```python
from build123d import *

# Parameters (mm, degrees)
SKETCH1_W           = 144
SKETCH1_H           = 331
BOSS_EXTRUDE1_DEPTH = 3
SKETCH2_R           = 5
CUT_EXTRUDE1_DEPTH  = 543.073379748
SKETCH3_R           = 5
CUT_EXTRUDE2_DEPTH  = 10
SKETCH4_R           = 5
CUT_EXTRUDE3_DEPTH  = 10
LPATTERN1_COUNT     = 4
LPATTERN1_PITCH     = 80
FILLET1_R           = 5


with BuildPart() as part:
    # Sketch1 → Boss-Extrude1 (new body)
    with BuildSketch(Plane.XY.offset(3)):
        with Locations((18.851179955, 368.89742901)):
            Rectangle(SKETCH1_W, SKETCH1_H)
    extrude(amount=-BOSS_EXTRUDE1_DEPTH)

    # Sketch2 → Cut-Extrude1 (cut, through all)
    with BuildSketch(Plane.XY.offset(3)):
        with Locations((63.851179955, 523.39742901)):
            Circle(SKETCH2_R)
        with Locations((64.635907686, 483.39742901)):
            Circle(SKETCH2_R)
        with Locations((64.635907686, 425.89742901)):
            Circle(SKETCH2_R)
        with Locations((64.635907686, 320.89742901)):
            Circle(SKETCH2_R)
        with Locations((64.635907686, 263.39742901)):
            Circle(SKETCH2_R)
        with Locations((64.635907686, 223.39742901)):
            Circle(SKETCH2_R)
    extrude(amount=-CUT_EXTRUDE1_DEPTH, mode=Mode.SUBTRACT)

    # Sketch3 → Cut-Extrude2 (cut)
    with BuildSketch(Plane.XY.offset(3)):
        with Locations((-26.148820045, 505.89742901)):
            Circle(SKETCH3_R)
        with Locations((-26.148820045, 400.89742901)):
            Circle(SKETCH3_R)
        with Locations((-26.148820045, 345.89742901)):
            Circle(SKETCH3_R)
        with Locations((-26.148820045, 240.89742901)):
            Circle(SKETCH3_R)
    extrude(amount=-CUT_EXTRUDE2_DEPTH, mode=Mode.SUBTRACT)

    # Sketch4 → Cut-Extrude3 (cut)
    with BuildSketch(Plane.XY.offset(3)):
        with Locations((-41.648820045, 253.39742901)):
            Circle(SKETCH4_R)
        with Locations((-11.148820045, 253.39742901)):
            Circle(SKETCH4_R)
        with Locations((48.851179955, 253.39742901)):
            Circle(SKETCH4_R)
        with Locations((79.351179955, 253.39742901)):
            Circle(SKETCH4_R)
    cut_extrude3 = extrude(amount=-CUT_EXTRUDE3_DEPTH, mode=Mode.SUBTRACT)

    # LPattern1: Cut-Extrude3 ×4
    with Locations(*[(0, i * LPATTERN1_PITCH, 0) for i in range(1, LPATTERN1_COUNT)]):
        add(cut_extrude3, mode=Mode.SUBTRACT)

    # Fillet1
    fillet1_edges = [part.edges().sort_by_distance(p)[0] for p in [
        (-53.148820045, 534.39742901, 1.5),
        (90.851179955, 534.39742901, 1.5),
    ]]
    fillet(fillet1_edges, radius=FILLET1_R)


solid = part.part
```
Can you work these out from the model? Positions are in its coordinate system, mm. Round coordinates to 2 decimals unless told otherwise and drop trailing zeros. Answer in a Markdown table with one row per item.
Item 1: Will this pin go through, and if not, where does the flat tip stop? P1, Ø6, axis at x = -11.15, y = 253.4, coming from the +Z side (3 decimals).
Answer block:
| item | result |
|---|---|
| P1 | through |
Item 2: Suppose I cut it at A-A, the plane z = 0.5. Give the number of separate pieces and of enclosed holes in the cut face, plus the area to 3 significant figures.
Answer block:
| item | result |
|---|---|
| separate pieces | 1 |
| enclosed holes | 26 |
| area | 45,600 mm² |
Item 3: If I drill on probe 1 along Y at (x, z) = (51, 2.25); probe 2 along Y at (x, z) = (48, 2.65); probe 3 along X at (y, z) = (259, 0.25), over which ranges is the centre line in solid material (lowest first)?
Answer block:
| item | result |
|---|---|
| probe 1 | 203.4 to 248.88, 257.91 to 328.88, 337.91 to 408.88, 417.91 to 488.88, 497.91 to 534.4 |
| probe 2 | 203.4 to 248.47, 258.32 to 328.47, 338.32 to 408.47, 418.32 to 488.47, 498.32 to 534.4 |
| probe 3 | -53.15 to 62.26, 67.02 to 90.85 |
Item 4: We'd pull the mould along Y, two halves only. Please class faces 1 (the flat face through (18, 371, 3)), 2 (the cylindrical face through (-38.961, 257.613, 1.521)): released by +Y, released by -Y, zero draft, split by the parting line, or undercut.
Answer block:
| item | result |
|---|---|
| face 1 | zero draft |
| face 2 | undercut |
